The listing builds one solid part. Answer for the finished solid, in the listing's coordinates (mm). Face numbers are marked on the shaded views. A direction names the side the tool comes from. Round coordinates to 2 decimals unless told otherwise and drop trailing zeros. Write each loop counter-clockwise with the first axis right and the second up, starting at its lowest first coordinate (ties: lowest second). Pieces come first, ordered by that corner, then holes. Notation, with made-up numbers: (-23.5, 11.5) - (26.5, 11.5) arc R12 cw to (26.5, 31.5) - close; hole circle Ø11 at (82, 12.5). An arc over 180 degrees is marked (long way). Answer in a Markdown table with one row per item.
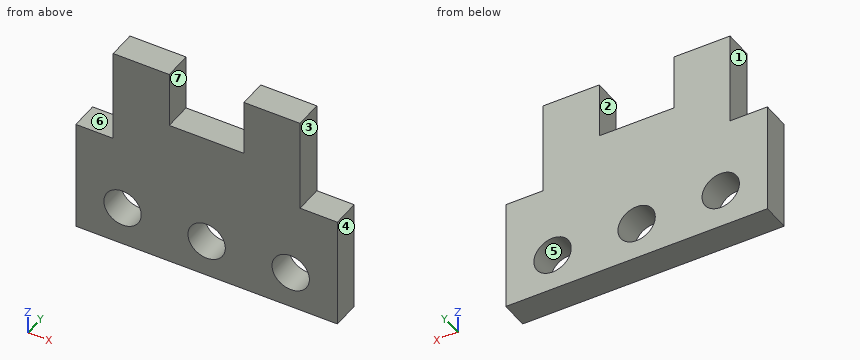
Autodesk Inventor part; units mm, degrees
ref_plane "YZ Plane" through (0, 0, 0) normal (1, 0, 0) x (0, 1, 0)
ref_plane "XZ Plane" through (0, 0, 0) normal (0, 1, 0) x (-1, 0, 0)
ref_plane "XY Plane" through (0, 0, 0) normal (0, 0, 1) x (1, 0, 0)
sketch "Sketch1" plane through (0, 0, 0) normal (0, 1, 0) x (-1, 0, 0)
  line L0 (0, 0) -> (0, 60)
  line L1 (0, 60) -> (20, 60)
  line L2 (20, 60) -> (20, 110)
  line L3 (20, 110) -> (50, 110)
  line L4 (50, 110) -> (50, 80)
  line L5 (50, 80) -> (90, 80)
  line L6 (90, 80) -> (90, 110)
  line L7 (90, 110) -> (120, 110)
  line L8 (120, 110) -> (120, 60)
  line L9 (120, 60) -> (140, 60)
  line L10 (140, 60) -> (140, 0)
  line L11 (140, 0) -> (0, 0)
  circle A0 centre (25, 20) radius 10
  circle A1 centre (70, 20) radius 10
  circle A2 centre (115, 21) radius 10
  dimension "d0" = 50
  dimension "d1" = 20
  dimension "d2" = 20
  dimension "d5" = 20
extrude "Extrusion1" add sketch "Sketch1" along normal blind 15
properties part number "P1-6"
(1) Section A-A (x = -25) is taken. Give the vertices of the cut face in (y, z).
Checked values:
| item | result |
|---|---|
| outline | (0, 0) - (15, 0) - (15, 10) - (0, 10) - close; (0, 30) - (15, 30) - (15, 110) - (0, 110) - close |
(2) Section D-D (x = -70) is taken. Give the vertices of the cut face in (y, z), and give its area (3 significant figures).
Checked values:
| item | result |
|---|---|
| outline | (0, 0) - (15, 0) - (15, 10) - (0, 10) - close; (0, 30) - (15, 30) - (15, 80) - (0, 80) - close |
| area | 900 mm2 |
(3) Flat-ended cylindrical pins translate along their axes: pin 1 (7.5 mm diameter, centred on x = -14, y = 9, fed in from +Z); pin 2 (3 mm diameter, centred on x = -52.5, y = 2.5, fed in from +Z). Find the tip coordinate at first contact, or state that the pin passes through.
Checked values:
| item | result |
|---|---|
| pin 1 | stops at z = 60 |
| pin 2 | stops at z = 80 |
(4) Section C-C (z = 28.5) is taken. Give the vertices of the cut face in (x, y).
Checked values:
| item | result |
|---|---|
| outline | (-140, 0) - (-121.61, 0) - (-121.61, 15) - (-140, 15) - close; (-108.39, 0) - (-75.27, 0) - (-75.27, 15) - (-108.39, 15) - close; (-64.73, 0) - (-30.27, 0) - (-30.27, 15) - (-64.73, 15) - close; (-19.73, 0) - (0, 0) - (0, 15) - (-19.73, 15) - close |
(5) For the marked faces 1, 2, 3 and 4, determine the directions among +Z, -Z, +X, -X, +Y, -Y from which every point of the face is accessible in a straight line to the end or side of a thin tool.
Checked values:
| item | result |
|---|---|
| face 1 | +Z, -X, +Y, -Y |
| face 2 | +Z, +Y, -Y |
| face 3 | +Z, +X, +Y, -Y |
| face 4 | +Z, -Z, +X, +Y, -Y |
(6) Section B-B (y = 3) is taken. Give the vertices of the cut face in (x, z), and give its area (3 significant figures).
Checked values:
| item | result |
|---|---|
| outline | (-140, 0) - (0, 0) - (0, 60) - (-20, 60) - (-20, 110) - (-50, 110) - (-50, 80) - (-90, 80) - (-90, 110) - (-120, 110) - (-120, 60) - (-140, 60) - close; hole circle Ø20 at (-115, 21); hole circle Ø20 at (-70, 20); hole circle Ø20 at (-25, 20) |
| area | 11,300 mm2 |
(7) Find the intervals of material crossed by line 1 (Z direction, x = -115, y = 7); line 2 (Z direction, x = -70, y = 4); line 3 (X direction, y = 6.75, z = 95), in increasing order.
Checked values:
| item | result |
|---|---|
| line 1 | z = 0 to 11, 31 to 110 |
| line 2 | z = 0 to 10, 30 to 80 |
| line 3 | x = -120 to -90, -50 to -20 |
(8) For a pull along Z with two mould halves and no side action, classify the marked faces 5, 6 and 7 as pulls with the +Z half, pulls with the -Z half, needs draft (parallel to the pull), parting line crosses it, or undercut.
Checked values:
| item | result |
|---|---|
| face 5 | undercut |
| face 6 | pulls with the +Z half |
| face 7 | needs draft |
